For this review, take the finished solid that the model builds, in its own axes (mm). A direction names the side the tool comes from. Coordinates: 2 decimals unless noted, no trailing zeros. Loops run counter-clockwise (first coordinate to the right, second up) from the corner with the lowest first, then second, coordinate; pieces in that order, holes last. Notation, with made-up numbers: (79, 71.5) - (105, 71.5) arc R18 cw to (105, 87.5) - close; hole circle Ø7 at (-37, -36.5). An arc over 180 degrees is marked (long way). One line per item, written item: value. Start each with the question number.
1. For faces 1 (the face through (1.323, -38.708, -10.074)), 2 (the face through (-32.234, -12.878, -15.132)), 3 (the face through (2.75, -46.94, 12.4)), list the 3-axis set-ups (+Z, -Z, +X, -X, +Y, -Y) from which the entire face can be reached by the end or side of a thin tool; tool diameter is ignored.
2. Take a section at A-A, the plane y = -12. State the section outline as (x, z) points.
3. Insertion check: pin 1 (4 mm diameter, centred on x = 24, z = -13.5, fed in from +Y); pin 2 (6 mm diameter, centred on x = 9.5, z = -19.5, fed in from -Y); pin 3 (1.5 mm diameter, centred on x = -5.5, y = -45, fed in from +Z). Each pin has a flat end and moves straight along its axis. Give the tip position at first contact, or say it passes through.
4. The part is to be moulded in two halves that separate along X. For faces 4 (the face through (-1, -11, -25.4)), 5 (the face through (31.756, -12.878, -12.421)), 6 (the face through (2.75, -30.43, 12.4)), say which applies: released by +X, released by -X, zero draft, split by the parting line, or undercut.
5. To check wall thickness, follow line 1 (Z direction, x = -38, y = -12); line 2 (X direction, y = -7, z = -12); line 3 (Y direction, x = 46, z = 12). State the ranges of each line that lie inside material, in increasing order. Write a range as from..to.
6. Take a section at B-B, the plane x = 38.1. State the section outline as (y, z) points.
```python
from build123d import *

# Parameters (mm, degrees)
F0_W     = 101.6
F0_H     = 50.8
F1_DEPTH = 25.4
F2_R     = 6.35
F3_DEPTH = 25.401
F4_W     = 12.7
F4_H     = 25.4
F6_W     = 6.9762246056
F6_H     = 6.35
F8_R     = 1.26999
F9_SIZE  = 2.54


# Not quite as in the source:
# - a fillet or chamfer is up to 0.001 mm smaller than in the source, because OpenCascade refuses the exact size


with BuildPart() as f1:
    # F0 (on Front) → F1 (new body)
    with BuildSketch(Plane.XZ):
        Rectangle(F0_W, F0_H)
    extrude(amount=F1_DEPTH)

    # F2 (on face) → F3 (cut, through all)
    with BuildSketch(Plane.XZ.offset(25.4)):
        with Locations((-38.1, 12.7)):
            Circle(F2_R)
        with Locations((-38.1, -12.7)):
            Circle(F2_R)
        with Locations((38.1, -12.7)):
            Circle(F2_R)
        with Locations((38.1, 12.7)):
            Circle(F2_R)
    extrude(amount=-F3_DEPTH, mode=Mode.SUBTRACT)

    # F4 (on Top) → F5 (revolve)
    with BuildSketch(Plane.XY):
        with Locations((-6.35, -38.1)):
            Rectangle(F4_W, F4_H)
    revolve(axis=Axis((0, -38.1, 0), (0, -1, 0)))

    # F6 (on Top) → F7 (revolve, cut)
    with BuildSketch(Plane.XY):
        with Locations((-13.6481123028, -38.735)):
            Rectangle(F6_W, F6_H)
    revolve(axis=Axis((0, -32.9395644367, 0), (0, -1, 0)), mode=Mode.SUBTRACT)

    # F8 (radius 1.27 in the source; OpenCascade refuses exactly that, so slightly less here)
    f8_edges = [f1.edges().sort_by_distance(p)[0] for p in [
        (12.7, -25.4, 0),
        (10.16, -41.91, 0),
        (10.16, -35.56, 0),
        (12.7, -41.91, 0),
        (12.7, -35.56, 0),
    ]]
    fillet(f8_edges, radius=F8_R)

    # F9
    f9_edges = [f1.edges().sort_by_distance(p)[0] for p in [
        (0, -25.4, -25.4),
        (-50.8, -25.4, 0),
        (0, -25.4, 25.4),
        (50.8, -25.4, 0),
    ]]
    chamfer(f9_edges, length=F9_SIZE)


solid = f1.part
```
Solutions:
1. face 1: none
1. face 2: +Y, -Y
1. face 3: -Y
2. outline: (-50.8, -25.4) - (50.8, -25.4) - (50.8, 25.4) - (-50.8, 25.4) - close; hole circle Ø12.7 at (-38.1, -12.7); hole circle Ø12.7 at (-38.1, 12.7); hole circle Ø12.7 at (38.1, -12.7); hole circle Ø12.7 at (38.1, 12.7)
3. pin 1: y = 0
3. pin 2: y = -25.4
3. pin 3: z = 11.78
4. face 4: zero draft
4. face 5: undercut
4. face 6: split by the parting line
5. line 1: -25.4..-19.05, -6.35..6.35, 19.05..25.4
5. line 2: -50.8..-44.41, -31.79..31.79, 44.41..50.8
5. line 3: -25.4..0
6. outline: (-25.4, -22.86) - (-22.86, -25.4) - (0, -25.4) - (0, -19.05) - (-25.4, -19.05) - close; (-25.4, -6.35) - (0, -6.35) - (0, 6.35) - (-25.4, 6.35) - close; (-25.4, 19.05) - (0, 19.05) - (0, 25.4) - (-22.86, 25.4) - (-25.4, 22.86) - close
